Input: part model. Units: mm. Frame: model coordinates. A direction names the side the tool comes from. Coordinates: 2 decimals unless noted, no trailing zeros. Write each loop counter-clockwise with the first axis right and the second up, starting at its lowest first coordinate (ties: lowest second). Pieces come first, ordered by that corner, then holes. Notation, with made-up numbers: (1, 2.5) - (9, 2.5) arc R32 cw to (9, 37.5) - close; hole circle Ø4 at (38, 44.5). An arc over 180 degrees is marked (long way). Use a Markdown table: item, result. Add a question column.
Q1. Section query A-A (z = 0). Return the cut outline in (x, y), then the cut area to 3 significant figures.
Q2. Pin query (flat end, axial travel): P1, Ø3, axis at x = -10.5, z = -13.5, coming from the +Y side; P2, Ø3, axis at x = -0.12, z = 15.02, coming from the -Y side; P3, Ø3, axis at y = 13, z = -15, coming from the -X side. Return the tip coordinate at first contact, or that it passes through.
Q3. Section query B-B (y = 20.25). Return the cut outline in (x, z).
Q4. Set-up query: faces 1 (the face through (15.57, 3.04, 14)), 2 (the face through (15, 6, 13)). Return all of +Z, -Z, +X, -X, +Y, -Y with unobstructed straight access to the full face (end or side cutting, diameter ignored); none if empty.
Q5. Section query D-D (z = 15.5). Return the cut outline in (x, y), then the cut area to 3 significant figures.
Q6. Material intervals for probe 1 along X at (y, z) = (6.5, 0); probe 2 along X at (y, z) = (3.5, 1.5); probe 3 along Y at (x, z) = (16.5, -11), sorted ascending. Write a range as from..to.
Q7. Mould query, pull axis Z, two halves, no side actions, for faces 3 (the face through (0, 10, -22)), 4 (the face through (0, 10, 22)), 5 (the face through (22, 10, 0)), 6 (the face through (-17.44, 13.18, -0.54)). Classes: released by +Z, released by -Z, zero draft, split by the parting line, or undercut.
Q8. Section query C-C (z = 7). Return the cut outline in (x, y).
from build123d import *
from build123d.topology import SkipClean

# Parameters (mm, degrees)
SKETCH1_W           = 44
SKETCH1_H           = 44
SKETCH1_R           = 1.5
BOSS_EXTRUDE1_DEPTH = 3
SKETCH2_W           = 44
SKETCH2_H           = 44
SKETCH2_W_2         = 36
SKETCH2_H_2         = 36
BOSS_EXTRUDE2_DEPTH = 20
SKETCH3_R           = 10.5
CUT_EXTRUDE1_DEPTH  = 20
SKETCH4_W           = 44
SKETCH4_H           = 44
BOSS_EXTRUDE3_DEPTH = 3
SKETCH5_R           = 10.5
CUT_EXTRUDE2_DEPTH  = 20
SKETCH6_R           = 10.5
BOSS_EXTRUDE4_DEPTH = 23
SKETCH7_R           = 2.5
CUT_EXTRUDE3_DEPTH  = 33
BOSS_EXTRUDE5_START = 3
SKETCH8_R           = 1.5
BOSS_EXTRUDE5_DEPTH = 3


with BuildPart() as part:
    # Sketch1 → Boss-Extrude1 (new body)
    with BuildSketch(Plane(origin=(0, 0, 0), x_dir=(1, 0, 0), z_dir=(0, 1, 0))):
        Rectangle(SKETCH1_W, SKETCH1_H)
        with Locations(Location((-15.5, 15.5, 0), (0, 0, 270))):
            Circle(SKETCH1_R, mode=Mode.SUBTRACT)
        with Locations(Location((15.5, 15.5, 0), (0, 0, 270))):
            Circle(SKETCH1_R, mode=Mode.SUBTRACT)
        with Locations(Location((-15.5, -15.5, 0), (0, 0, 270))):
            Circle(SKETCH1_R, mode=Mode.SUBTRACT)
        with Locations(Location((15.5, -15.5, 0), (0, 0, 270))):
            Circle(SKETCH1_R, mode=Mode.SUBTRACT)
    extrude(amount=BOSS_EXTRUDE1_DEPTH)

    # Sketch2 → Boss-Extrude2 (add)
    with BuildSketch(Plane(origin=(0, 3, 0), x_dir=(1, 0, 0), z_dir=(0, 1, 0))):
        Rectangle(SKETCH2_W, SKETCH2_H)
        Rectangle(SKETCH2_W_2, SKETCH2_H_2, mode=Mode.SUBTRACT)
    extrude(amount=BOSS_EXTRUDE2_DEPTH)

    # Sketch3 → Cut-Extrude1 (cut)
    with BuildSketch(Plane(origin=(0, 3, 0), x_dir=(1, 0, 0), z_dir=(0, 1, 0))):
        with Locations(Location((0, 0, 0), (0, 0, 270))):
            Circle(SKETCH3_R)
    extrude(amount=-CUT_EXTRUDE1_DEPTH, mode=Mode.SUBTRACT)

    # Sketch4 → Boss-Extrude3 (add)
    with BuildSketch(Plane(origin=(0, 23, 0), x_dir=(1, 0, 0), z_dir=(0, 1, 0))):
        Rectangle(SKETCH4_W, SKETCH4_H)
    extrude(amount=BOSS_EXTRUDE3_DEPTH)

    # Sketch5 → Cut-Extrude2 (cut)
    with BuildSketch(Plane(origin=(0, 26, 0), x_dir=(1, 0, 0), z_dir=(0, 1, 0))):
        with Locations(Location((0, 0, 0), (0, 0, 270))):
            Circle(SKETCH5_R)
        with BuildLine():
            Line((-22, 22), (-22, 19.241657387))
            ThreePointArc((-22, 19.241657387), (-10.196699141, 10.196699141), (-19.241657387, 22))
            Line((-19.241657387, 22), (-22, 22))
        make_face()
        with BuildLine():
            Line((22, 22), (19.241657387, 22))
            ThreePointArc((19.241657387, 22), (10.196699141, 10.196699141), (22, 19.241657387))
            Line((22, 19.241657387), (22, 22))
        make_face()
        with BuildLine():
            Line((22, -22), (22, -19.241657387))
            ThreePointArc((22, -19.241657387), (10.196699141, -10.196699141), (19.241657387, -22))
            Line((19.241657387, -22), (22, -22))
        make_face()
        with BuildLine():
            Line((-22, -22), (-22, -19.241657387))
            ThreePointArc((-22, -19.241657387), (-10.196699141, -10.196699141), (-19.241657387, -22))
            Line((-19.241657387, -22), (-22, -22))
        make_face()
    extrude(amount=-CUT_EXTRUDE2_DEPTH, mode=Mode.SUBTRACT)

    # Sketch6 → Boss-Extrude4 (add)
    with SkipClean():  # the faces are left unmerged after this step: merging them gives an invalid solid
        with BuildSketch(Plane.XZ.offset(-23)):
            with BuildLine():
                Line((8.428932188, 18), (-8.428932188, 18))
                ThreePointArc((-8.428932188, 18), (-10.196699141, 10.196699141), (-18, 8.428932188))
                Line((-18, 8.428932188), (-18, -8.428932188))
                ThreePointArc((-18, -8.428932188), (-10.196699141, -10.196699141), (-8.428932188, -18))
                Line((-8.428932188, -18), (8.428932188, -18))
                ThreePointArc((8.428932188, -18), (10.196699141, -10.196699141), (18, -8.428932188))
                Line((18, -8.428932188), (18, 8.428932188))
                ThreePointArc((18, 8.428932188), (10.196699141, 10.196699141), (8.428932188, 18))
            make_face()
            with Locations(Location((0, 0, 0), (0, 0, 90))):
                Circle(SKETCH6_R, mode=Mode.SUBTRACT)
        extrude(amount=BOSS_EXTRUDE4_DEPTH)

    # Sketch7 → Cut-Extrude3 (cut)
    with SkipClean():  # the faces are left unmerged after this step: merging them gives an invalid solid
        with BuildSketch(Plane(origin=(0, 26, 0), x_dir=(1, 0, 0), z_dir=(0, 1, 0))):
            with Locations(Location((15, 0, 0), (0, 0, 270))):
                Circle(SKETCH7_R)
            with Locations(Location((-15, 0, 0), (0, 0, 270))):
                Circle(SKETCH7_R)
            with Locations(Location((-0.695414312, 14.983871293, 0), (0, 0, 270))):
                Circle(SKETCH7_R)
            with Locations(Location((-0.115302399, -15.016128707, 0), (0, 0, 270))):
                Circle(SKETCH7_R)
        extrude(amount=-CUT_EXTRUDE3_DEPTH, mode=Mode.SUBTRACT)

    # Sketch8 → Boss-Extrude5 (add)
    # profile 1 of 4: a face of its own
    with SkipClean():  # the faces are left unmerged after this step: merging them gives an invalid solid
        with BuildSketch(Plane(origin=(0, 3, 0), x_dir=(1, 0, 0), z_dir=(0, 1, 0)).offset(BOSS_EXTRUDE5_START)):
            with BuildLine():
                Line((8.428932188, -18), (18, -18))
                Line((18, -18), (18, -8.428932188))
                ThreePointArc((18, -8.428932188), (10.196699141, -10.196699141), (8.428932188, -18))
            make_face()
            with Locations(Location((15.5, -15.5, 0), (0, 0, 270))):
                Circle(SKETCH8_R, mode=Mode.SUBTRACT)
        # profile 2 of 4: a face of its own
        with BuildSketch(Plane(origin=(0, 3, 0), x_dir=(1, 0, 0), z_dir=(0, 1, 0)).offset(BOSS_EXTRUDE5_START)):
            with BuildLine():
                Line((18, 8.428932188), (18, 18))
                Line((18, 18), (8.428932188, 18))
                ThreePointArc((8.428932188, 18), (10.196699141, 10.196699141), (18, 8.428932188))
            make_face()
            with Locations(Location((15.5, 15.5, 0), (0, 0, 270))):
                Circle(SKETCH8_R, mode=Mode.SUBTRACT)
        # profile 3 of 4: a face of its own
        with BuildSketch(Plane(origin=(0, 3, 0), x_dir=(1, 0, 0), z_dir=(0, 1, 0)).offset(BOSS_EXTRUDE5_START)):
            with BuildLine():
                Line((-8.428932188, 18), (-18, 18))
                Line((-18, 18), (-18, 8.428932188))
                ThreePointArc((-18, 8.428932188), (-10.196699141, 10.196699141), (-8.428932188, 18))
            make_face()
            with Locations(Location((-15.5, 15.5, 0), (0, 0, 270))):
                Circle(SKETCH8_R, mode=Mode.SUBTRACT)
        # profile 4 of 4: a face of its own
        with BuildSketch(Plane(origin=(0, 3, 0), x_dir=(1, 0, 0), z_dir=(0, 1, 0)).offset(BOSS_EXTRUDE5_START)):
            with BuildLine():
                Line((-18, -8.428932188), (-18, -18))
                Line((-18, -18), (-8.428932188, -18))
                ThreePointArc((-8.428932188, -18), (-10.196699141, -10.196699141), (-18, -8.428932188))
            make_face()
            with Locations(Location((-15.5, -15.5, 0), (0, 0, 270))):
                Circle(SKETCH8_R, mode=Mode.SUBTRACT)
        extrude(amount=-BOSS_EXTRUDE5_DEPTH)


solid = part.part
Values follow:
| question | item | result |
|---|---|---|
| 1 | outline | (-22, 0) - (-17.5, 0) - (-17.5, 26) - (-22, 26) - close; (-12.5, 0) - (-10.5, 0) - (-10.5, 26) - (-12.5, 26) - close; (10.5, 0) - (12.5, 0) - (12.5, 26) - (10.5, 26) - close; (17.5, 0) - (22, 0) - (22, 26) - (17.5, 26) - close |
| 1 | area | 338 mm2 |
| 2 | P1 | y = 6 |
| 2 | P2 | through |
| 2 | P3 | x = -8.27 |
| 3 | outline | (-22, -11.76) arc R7.5 cw (long way) to (-11.76, -22) - (11.76, -22) arc R7.5 cw (long way) to (22, -11.76) - (22, 11.76) arc R7.5 cw (long way) to (11.76, 22) - (-11.76, 22) arc R7.5 cw (long way) to (-22, 11.76) - close; hole circle Ø5 at (-15, 0); hole circle Ø21 at (0, 0); hole circle Ø5 at (-0.7, -14.98); hole circle Ø5 at (-0.12, 15.02); hole circle Ø5 at (15, 0) |
| 4 | face 1 | +Y, -Y |
| 4 | face 2 | +Y |
| 5 | outline | (-22, 0) - (-17, 0) - (-17, 6) - (-22, 6) - close; (-14, 0) - (-2.57, 0) - (-2.57, 26) - (-8, 26) - (-8, 6) - (-14, 6) - close; (2.34, 0) - (14, 0) - (14, 6) - (8, 6) - (8, 26) - (2.34, 26) - close; (17, 0) - (22, 0) - (22, 6) - (17, 6) - close |
| 5 | area | 420 mm2 |
| 6 | probe 1 | -22..-17.5, -12.5..-10.5, 10.5..12.5, 17.5..22 |
| 6 | probe 2 | -22..-17, -13..-10.39, 10.39..13, 17..22 |
| 6 | probe 3 | 0..6 |
| 7 | face 3 | released by -Z |
| 7 | face 4 | released by +Z |
| 7 | face 5 | zero draft |
| 7 | face 6 | undercut |
| 8 | outline | (-22, 0) - (-7.83, 0) - (-7.83, 26) - (-22, 26) - close; (7.83, 0) - (22, 0) - (22, 26) - (7.83, 26) - close |
